Could you check a few things on this drawing? It's one solid part, dimensions in mm from its lowest x, y, z. A direction names the side the tool comes from. Round coordinates to 2 decimals unless told otherwise and drop trailing zeros. Loops run counter-clockwise (first coordinate to the right, second up) from the corner with the lowest first, then second, coordinate; pieces in that order, holes last. Notation, with made-up numbers: M 61.5,53 L 77.5,53 A16 cw 77.5,63 Z; hole C 31,80.5 d5. An arc over 180 degrees is marked long. Answer as a JSON object with one key per item and string values.
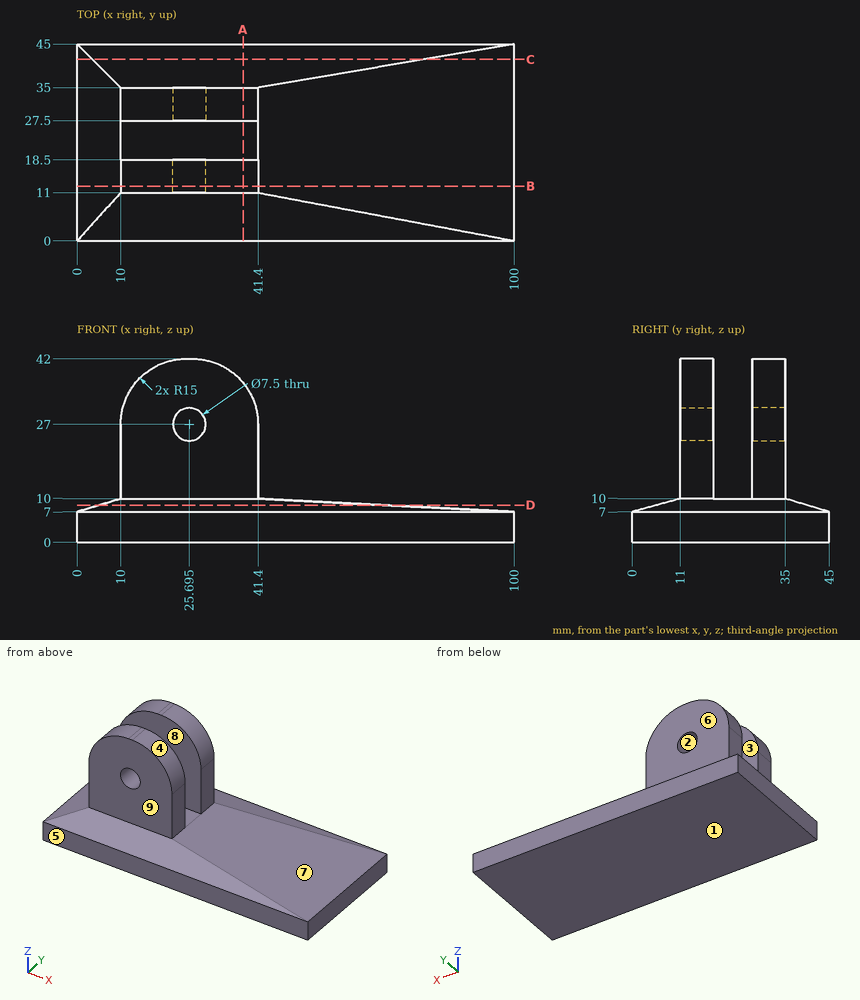
Item 1: I'm going to push flat-ended pins straight in: pin 1 Ø6 at (y, z) = (16.5, 15) entering from -X; pin 2 Ø7 at (x, y) = (33, 21) entering from +Z; pin 3 Ø2 at (y, z) = (27, 14) entering from +X; pin 4 Ø4.5 at (x, z) = (25.69, 27) entering from -Y. Where does each tip first touch, or does it pass through?
Resolved:
{"pin 1": "x = 10", "pin 2": "z = 41.41", "pin 3": "x = 41.4", "pin 4": "through"}
Item 2: If we mould it in two halves opening along Z, with no side actions, what happens to the marked faces 1, 2, 3 and 4? For each: pulls with the +Z half, pulls with the -Z half, needs draft (parallel to the pull), parting line crosses it, or undercut.
Resolved:
{"face 1": "pulls with the -Z half", "face 2": "undercut", "face 3": "needs draft", "face 4": "pulls with the +Z half"}
Item 3: I want a section at A-A, the plane x = 38. Please give me the cut outline in (y, z), then the cut area to 3 significant figures.
Resolved:
{"outline": "M 0,0 L 45,0 L 45,7 L 35,10 L 35,36.51 L 27.5,36.51 L 27.5,10 L 18.5,10 L 18.5,36.51 L 11,36.51 L 11,10 L 0,7 Z", "area": "816 mm²"}
Item 4: I want a section at C-C, the plane y = 41.5. Please give me the cut outline in (x, z), then the cut area to 3 significant figures.
Resolved:
{"outline": "M 0,0 L 100,0 L 100,7 L 79.49,8.05 L 3.5,8.05 L 0,7 Z", "area": "792 mm²"}
Item 5: On a 3-axis mill with a long thin cutter (end or side, diameter ignored), from which of +Z, -Z, +X, -X, +Y, -Y can I reach the whole of each face in a straight line? I mean the marked faces 5, 6, 7, 8 and 9. Say none if no direction works.
Resolved:
{"face 5": "+Z, -Z, +X, -X, -Y", "face 6": "+Z, +X, -X, +Y", "face 7": "+Z, +X, +Y, -Y", "face 8": "+Z, +X, -X", "face 9": "+Z, +X, -X, -Y"}
Item 6: I want a section at B-B, the plane y = 12.5. Please give me the cut outline in (x, z) (3 decimals).
Resolved:
{"outline": "M 0,0 L 100,0 L 100,7 L 41.4,10 L 41.4,27 A15 ccw 26.4,42 L 25,42 A15 ccw 10,27 L 10,10 L 0,7 Z; hole C 25.695,27 d7.5"}
Item 7: Please list where these lines run through material, in increasing order: probe 1 along Y at (x, z) = (38, 15); probe 2 along X at (y, z) = (16, 27) (3 decimals); probe 3 along Z at (x, y) = (29, 25.5). Write a range as from..to.
Resolved:
{"probe 1": "11..18.5, 27.5..35", "probe 2": "10..21.945, 29.445..41.4", "probe 3": "0..10"}
Item 8: I want a section at D-D, the plane z = 8.5. Please give me the cut outline in (x, y), then the cut area to 3 significant figures.
Resolved:
{"outline": "M 5,5.5 L 70.7,5.5 L 70.7,40 L 5,40 Z", "area": "2,270 mm²"}
